Can you work these out from the model? Positions are in its coordinate system, mm. Give positions to 0.01 mm unless a question says otherwise; leave off trailing zeros. Order: outer loops, then holes, each group sorted by start corner. A loop starts at its lowest first (then second) coordinate and runs counter-clockwise, first axis right, second up. Notation, with made-up numbers: M -15.5,-16 L 22.5,-16 A18 cw 22.5,-6 Z; hole C 55,31.5 d10. An arc over 180 degrees is marked long. Answer as a JSON object with one key per item and string values.
```python
from build123d import *

# Parameters (mm, degrees)
BOSS_EXTRUDE1_OUTLINE_R = 55.125
BOSS_EXTRUDE1_DEPTH     = 10
FILLET1_R               = 50
SKETCH4_R               = 2
CUT_EXTRUDE1_DEPTH      = 1336.164989569
SKETCH5_R               = 4.1
CUT_EXTRUDE2_DEPTH      = 1336.164989569


# Read off the part's stored shape, not the designer's step: Boss-Extrude1
with BuildPart() as part:
    # Boss-Extrude1 outline → Boss-Extrude1 (new body)
    with BuildSketch(Plane.ZY.offset(-1.65)):
        with BuildLine():
            Line((-1257.876937074, 266.919395505), (-1129.454602927, 237.627573392))
            ThreePointArc((-1129.454602927, 237.627573392), (-1096.744938567, 238.616085951), (-1068.662335154, 255.416880135))
            Line((-1068.662335154, 255.416880135), (-986.642796778, 338.794101601))
            ThreePointArc((-986.642796778, 338.794101601), (-984.910512742, 346.53132054), (-991.089695369, 351.499526147))
            Line((-991.089695369, 351.499526147), (-1086.722744118, 363.055830047))
            Line((-1086.722744118, 363.055830047), (-1159.562924749, 428.883221767))
            ThreePointArc((-1159.562924749, 428.883221767), (-1167.409525964, 430.269317516), (-1172.0754788, 423.810269894))
            Line((-1172.0754788, 423.810269894), (-1177.78637409, 336.842019695))
            Line((-1177.78637409, 336.842019695), (-1260.437346066, 280.42610587))
            ThreePointArc((-1260.437346066, 280.42610587), (-1263.57786788, 272.834732614), (-1257.876937074, 266.919395505))
        make_face()
        with Locations((-1115, 301)):
            Circle(BOSS_EXTRUDE1_OUTLINE_R, mode=Mode.SUBTRACT)
    extrude(amount=BOSS_EXTRUDE1_DEPTH)

    # Fillet1
    fillet1_edges = [part.edges().sort_by_distance(p)[0] for p in [
        (-3.35, 336.842019695, -1177.78637409),
        (-3.35, 363.055830047, -1086.722744118),
    ]]
    fillet(fillet1_edges, radius=FILLET1_R)

    # Sketch4 → Cut-Extrude1 (cut, through all)
    with BuildSketch(Plane.ZY.offset(-1.65)):
        with Locations((-1062.930222597, 331.0625)):
            Circle(SKETCH4_R)
        with Locations((-1115, 361.125)):
            Circle(SKETCH4_R)
        with Locations((-1062.930222597, 270.9375)):
            Circle(SKETCH4_R)
        with Locations((-1115, 240.875)):
            Circle(SKETCH4_R)
        with Locations((-1167.069777403, 270.9375)):
            Circle(SKETCH4_R)
        with Locations((-1167.069777403, 331.0625)):
            Circle(SKETCH4_R)
    extrude(amount=CUT_EXTRUDE1_DEPTH, mode=Mode.SUBTRACT)

    # Sketch5 → Cut-Extrude2 (cut, through all)
    with BuildSketch(Plane.ZY.offset(-1.65)):
        with Locations((-1164.591596996, 423.318830027)):
            Circle(SKETCH5_R)
        with Locations((-991.989450415, 344.053692355)):
            Circle(SKETCH5_R)
        with Locations((-1256.209098275, 274.231598575)):
            Circle(SKETCH5_R)
    extrude(amount=CUT_EXTRUDE2_DEPTH, mode=Mode.SUBTRACT)


solid = part.part
```
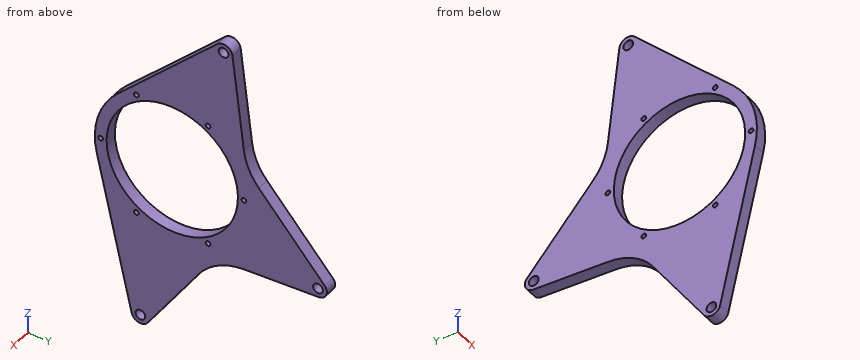
1) I need wall thicknesses on L1, parallel to Z at x = -1.75, y = 341.5; L2, parallel to Y at x = -2.5, z = -1115 (3 decimals); L3, parallel to Y at x = 0.75, z = -1085. Which ranges of each line are inside material? Lowest first, please.
Results found:
{"L1": "z = -1181.64 to -1152.4, -1077.6 to -995.2, -988.78 to -984.94", "L2": "y = 236 to 238.875, 242.875 to 245.875, 356.125 to 359.125, 363.125 to 388.611", "L3": "y = 243.34 to 254.75, 347.25 to 364.98"}
2) I want a section at B-B on x = -6.75. Count the separate pieces of the cut face and the enclosed holes in it, and give its area (3 significant figures).
Results found:
{"separate pieces": "1", "enclosed holes": "10", "area": "15,900 mm²"}
3) I want a section at C-C on y = 379.5. Write out the boundary of the cut face in (x, z), and give its area (3 significant figures).
Results found:
{"outline": "M -8.35,-1174.99 L 1.65,-1174.99 L 1.65,-1104.92 L -8.35,-1104.92 Z", "area": "701 mm²"}
4) I want a section at A-A on y = 301. Write out the boundary of the cut face in (x, z) (3 decimals), and give its area (3 significant figures).
Results found:
{"outline": "M -8.35,-1230.296 L 1.65,-1230.296 L 1.65,-1170.125 L -8.35,-1170.125 Z; M -8.35,-1059.875 L 1.65,-1059.875 L 1.65,-1023.821 L -8.35,-1023.821 Z", "area": "962 mm²"}
5) I'm going to push flat-ended pins straight in: pin 1 Ø1 at (x, z) = (-3, -1212) entering from -Y; pin 2 Ø2 at (x, y) = (-5, 285.5) entering from +Z; pin 3 Ø1.5 at (x, y) = (-3, 333.5) entering from -Z; pin 4 Ø2.5 at (y, z) = (361.125, -1115) entering from -X. Where does each tip first touch, or does it pass through?
Results found:
{"pin 1": "stops at y = 256.34", "pin 2": "stops at z = -1038.09", "pin 3": "stops at z = -1187.39", "pin 4": "passes through"}
6) I want a section at D-D on z = -1023. Write out the boundary of the cut face in (x, y).
Results found:
{"outline": "M -8.35,301.84 L 1.65,301.84 L 1.65,355.36 L -8.35,355.36 Z"}
